CAD build for the part. Positions are in the model's coordinates, mm. A direction names the side the tool comes from. Give positions to 0.01 mm unless a question says otherwise; leave off trailing zeros. Loops run counter-clockwise (first coordinate to the right, second up) from the corner with the lowest first, then second, coordinate; pieces in that order, holes last.
```python
from build123d import *

# Parameters (mm, degrees)
SKETCH1_W                  = 323.85
SKETCH1_H                  = 101.6
EXTRUDE1_DEPTH             = 6.35
SKETCH2_W                  = 57.15
SKETCH2_H                  = 76.2
CUT_EXTRUDE1_DEPTH         = 6.35
SKETCH3_W                  = 60.325
SKETCH3_H                  = 76.2
SKETCH3_W_2                = 50.8
SKETCH3_W_3                = 117.475
CUT_EXTRUDE2_DEPTH         = 6.35
SKETCH4_W                  = 6.35
SKETCH4_H                  = 6.35
CUT_EXTRUDE3_DEPTH         = 6.35
F_2_CLEARANCE_HOLE1_D      = 2.4384
FILLET1_R                  = 3.175
TAP_DRILL_FOR_8_TAP1_D     = 3.4544
TAP_DRILL_FOR_8_TAP1_DEPTH = 12.7
TAP_DRILL_FOR_8_TAP1_TIP   = 1.037806461
F_6_CLEARANCE_HOLE1_D      = 3.7973
F_6_CLEARANCE_HOLE1_DEPTH  = 12.7
F_6_CLEARANCE_HOLE1_TIP    = 1.140824014
TAP_DRILL_FOR_6_TAP1_D     = 2.7051
TAP_DRILL_FOR_6_TAP1_DEPTH = 12.7
TAP_DRILL_FOR_6_TAP1_TIP   = 0.81269403
FILLET2_R                  = 6.35
FILLET3_R                  = 6.35
TAP_DRILL_FOR_6_TAP2_D     = 2.7051
TAP_DRILL_FOR_6_TAP2_DEPTH = 101.6
TAP_DRILL_FOR_6_TAP2_TIP   = 0.81269403
TAP_DRILL_FOR_4_TAP1_D     = 2.2606


with BuildPart() as part:
    # Sketch1 → Extrude1 (new body)
    with BuildSketch(Plane(origin=(0, 0, 0), x_dir=(1, 0, 0), z_dir=(0, 1, 0))):
        Rectangle(SKETCH1_W, SKETCH1_H)
    extrude(amount=EXTRUDE1_DEPTH)

    # Sketch2 → Cut-Extrude1 (cut)
    with BuildSketch(Plane(origin=(0, 6.35, 0), x_dir=(-1, 0, 0), z_dir=(0, 1, 0))):
        with Locations((133.35, 0)):
            Rectangle(SKETCH2_W, SKETCH2_H)
    extrude(amount=-CUT_EXTRUDE1_DEPTH, mode=Mode.SUBTRACT)

    # Sketch3 → Cut-Extrude2 (cut)
    with BuildSketch(Plane(origin=(0, 6.35, 0), x_dir=(-1, 0, 0), z_dir=(0, 1, 0))):
        with Locations((61.9125, 0)):
            Rectangle(SKETCH3_W, SKETCH3_H)
        with Locations((-136.525, 0)):
            Rectangle(SKETCH3_W_2, SKETCH3_H)
        with Locations((-39.6875, 0)):
            Rectangle(SKETCH3_W_3, SKETCH3_H)
    extrude(amount=-CUT_EXTRUDE2_DEPTH, mode=Mode.SUBTRACT)

    # Sketch4 → Cut-Extrude3 (cut)
    with BuildSketch(Plane(origin=(0, 6.35, 0), x_dir=(-1, 0, 0), z_dir=(0, 1, 0))):
        with Locations((-158.75, -44.45)):
            Rectangle(SKETCH4_W, SKETCH4_H)
        with Locations((-158.75, 44.45)):
            Rectangle(SKETCH4_W, SKETCH4_H)
    extrude(amount=-CUT_EXTRUDE3_DEPTH, mode=Mode.SUBTRACT)

    # #2 Clearance Hole1 (through all)
    with Locations(Plane(origin=(158.75, 3.175, 50.8), x_dir=(1, 0, 0), z_dir=(0, 0, 1))):
        with Locations((0, 0)):
            Hole(F_2_CLEARANCE_HOLE1_D / 2)

    # Fillet1
    fillet1_edges = [part.edges().sort_by_distance(p)[0] for p in [
        (161.925, 6.35, 49.2125),
        (161.925, 6.35, -39.6875),
        (161.925, 6.35, -49.2125),
        (161.925, 6.35, 39.6875),
    ]]
    fillet(fillet1_edges, radius=FILLET1_R)

    # Tap Drill for #8 Tap1
    with Locations(Plane(origin=(-98.425, 6.35, -19.05), x_dir=(0, 0, 1), z_dir=(0, 1, 0))):
        with Locations((0, 0)):
            Hole(TAP_DRILL_FOR_8_TAP1_D / 2, depth=TAP_DRILL_FOR_8_TAP1_DEPTH)
            with Locations((0, 0, -(TAP_DRILL_FOR_8_TAP1_DEPTH + TAP_DRILL_FOR_8_TAP1_TIP / 2))):  # 118° drill point
                Cone(0, TAP_DRILL_FOR_8_TAP1_D / 2, TAP_DRILL_FOR_8_TAP1_TIP, mode=Mode.SUBTRACT)

    # #6 Clearance Hole1
    with Locations(Plane(origin=(-25.4, 6.35, -44.45), x_dir=(0, 0, 1), z_dir=(0, 1, 0))):
        with Locations((0, 0), (88.9, 0)):
            Hole(F_6_CLEARANCE_HOLE1_D / 2, depth=F_6_CLEARANCE_HOLE1_DEPTH)
            with Locations((0, 0, -(F_6_CLEARANCE_HOLE1_DEPTH + F_6_CLEARANCE_HOLE1_TIP / 2))):  # 118° drill point
                Cone(0, F_6_CLEARANCE_HOLE1_D / 2, F_6_CLEARANCE_HOLE1_TIP, mode=Mode.SUBTRACT)

    # Tap Drill for #6 Tap1
    with Locations(Plane(origin=(-149.225, 6.35, -44.45), x_dir=(0, 0, 1), z_dir=(0, 1, 0))):
        with Locations((0, 0), (88.9, 0)):
            Hole(TAP_DRILL_FOR_6_TAP1_D / 2, depth=TAP_DRILL_FOR_6_TAP1_DEPTH)
            with Locations((0, 0, -(TAP_DRILL_FOR_6_TAP1_DEPTH + TAP_DRILL_FOR_6_TAP1_TIP / 2))):  # 118° drill point
                Cone(0, TAP_DRILL_FOR_6_TAP1_D / 2, TAP_DRILL_FOR_6_TAP1_TIP, mode=Mode.SUBTRACT)

    # Fillet2
    fillet2_edges = [part.edges().sort_by_distance(p)[0] for p in [
        (-104.775, 3.175, -38.1),
        (-104.775, 3.175, 38.1),
        (-92.075, 3.175, 38.1),
        (-92.075, 3.175, -38.1),
        (-31.75, 3.175, -38.1),
        (-31.75, 3.175, 38.1),
        (111.125, 3.175, 38.1),
        (111.125, 3.175, -38.1),
    ]]
    fillet(fillet2_edges, radius=FILLET2_R)

    # Fillet3
    fillet3_edges = [part.edges().sort_by_distance(p)[0] for p in [
        (-19.05, 3.175, 38.1),
        (-19.05, 3.175, -38.1),
        (98.425, 3.175, -38.1),
        (98.425, 3.175, 38.1),
    ]]
    fillet(fillet3_edges, radius=FILLET3_R)

    # Tap Drill for #6 Tap2
    with Locations(Plane(origin=(60.325, 0, 44.45), x_dir=(0, 0, -1), z_dir=(0, -1, 0))):
        with Locations((0, 0), (0, 25.4), (88.9, 0), (88.9, 25.4)):
            Hole(TAP_DRILL_FOR_6_TAP2_D / 2, depth=TAP_DRILL_FOR_6_TAP2_DEPTH)
            with Locations((0, 0, -(TAP_DRILL_FOR_6_TAP2_DEPTH + TAP_DRILL_FOR_6_TAP2_TIP / 2))):  # 118° drill point
                Cone(0, TAP_DRILL_FOR_6_TAP2_D / 2, TAP_DRILL_FOR_6_TAP2_TIP, mode=Mode.SUBTRACT)

    # Tap Drill for #4 Tap1 (through all)
    with Locations(Plane(origin=(104.775, 6.35, 14.478), x_dir=(0, 0, 1), z_dir=(0, 1, 0))):
        with Locations((0, 0), (-28.956, 0)):
            Hole(TAP_DRILL_FOR_4_TAP1_D / 2)


solid = part.part
```
1. Saw through at B-B, the plane z = 6. List the corners of the cut face in (x, y) (3 decimals).
Responses:
outline: (-104.775, 0) - (-92.075, 0) - (-92.075, 6.35) - (-104.775, 6.35) - close; (-31.75, 0) - (-19.05, 0) - (-19.05, 6.35) - (-31.75, 6.35) - close; (98.425, 0) - (111.125, 0) - (111.125, 6.35) - (98.425, 6.35) - close
2. Saw through at A-A, the plane x = 25. List the corners of the cut face in (y, z).
Responses:
outline: (0, -50.8) - (6.35, -50.8) - (6.35, -38.1) - (0, -38.1) - close; (0, 38.1) - (6.35, 38.1) - (6.35, 50.8) - (0, 50.8) - close
3. Pull direction Z, two halves, no side cores. Call faces 5 (the face through (113.035, 3.131, -36.289)), 6 (the face through (-26, 6.35, 4)): released by +Z, released by -Z, zero draft, split by the parting line, or undercut.
Responses:
face 5: undercut
face 6: zero draft
4. Drop flat-ended pins along their axis: pin 1 (5 mm diameter, centred on x = -25.4, z = -44.45, fed in from +Y); pin 2 (1.9 mm diameter, centred on y = 3, z = -44.5, fed in from +X) (3 decimals). Give the stop position or say it passes through.
Responses:
pin 1: stops at y = 6.35
pin 2: stops at x = 155.575
5. Tool access for faces 1 (the face through (96.614, 3.131, 36.19)), 2 (the face through (-104.775, 3, 0)), 3 (the face through (155.575, 3, -44)), 4 (the face through (-161.925, 3, -44)): list every direction of +Z, -Z, +X, -X, +Y, -Y with a clear straight run to the whole face (end or side of a thin tool).
Responses:
face 1: +Y, -Y
face 2: -X, +Y, -Y
face 3: +X, +Y, -Y
face 4: +Z, -Z, -X, +Y, -Y
6. Probe line 1 along X through (y, z) = (1.25, -6) (3 decimals); line 2 along X through (y, z) = (3.25, -44.45) (3 decimals); line 3 along Z through (x, y) = (81.5, 5.5). List the from-to ranges inside material, lowest first.
Responses:
line 1: x = -104.775 to -92.075, -31.75 to -19.05, 98.425 to 111.125
line 2: x = -161.925 to -150.578, -147.872 to -27.299, -23.501 to 58.972, 61.678 to 84.372, 87.078 to 155.575
line 3: z = -50.8 to -38.1, 38.1 to 50.8
